from build123d import *

# Parameters (mm, degrees)
F1_DEPTH = 7.62
F2_R     = 2.54
F3_DEPTH = 25.4
F4_R     = 19.05
F4_R_2   = 8.89
F5_DEPTH = 25.4


with BuildPart() as f1:
    # F0 (on Top) → F1 (new body)
    with BuildSketch(Plane.XY):
        with BuildLine():
            ThreePointArc((-279.9174020173, 43.9496934414), (-263.0302165533, 39.4233371805), (-253.0018394569, 53.7445308008))
            ThreePointArc((-253.0018394569, 53.7445308008), (-262.5723411754, 67.8907101167), (-279.2635703278, 64.2696934414))
            Line((-279.2635703278, 64.2696934414), (-279.2635703278, 43.9496934414))
            Line((-279.2635703278, 43.9496934414), (-279.9174020173, 43.9496934414))
        make_face()
        with BuildLine():
            Line((-279.2635703278, 43.9496934414), (-279.2635703278, 64.2696934414))
            ThreePointArc((-279.2635703278, 64.2696934414), (-283.4739562591, 54.2346509123), (-279.9174020173, 43.9496934414))
            Line((-279.9174020173, 43.9496934414), (-279.2635703278, 43.9496934414))
        make_face()
        with BuildLine():
            ThreePointArc((-279.9174020173, 43.9496934414), (-283.4739562591, 54.2346509123), (-279.2635703278, 64.2696934414))
            Line((-279.2635703278, 64.2696934414), (-373.075891919, 64.2696934414))
            ThreePointArc((-373.075891919, 64.2696934414), (-370.1983304941, 59.5476620895), (-369.1951172447, 54.1096934414))
            ThreePointArc((-369.1951172447, 54.1096934414), (-370.1983304941, 48.6717247932), (-373.075891919, 43.9496934414))
            Line((-373.075891919, 43.9496934414), (-279.9174020173, 43.9496934414))
        make_face()
        with BuildLine():
            ThreePointArc((-369.1951172447, 54.1096934414), (-370.1983304941, 59.5476620895), (-373.075891919, 64.2696934414))
            Line((-373.075891919, 64.2696934414), (-373.2435703278, 64.2696934414))
            Line((-373.2435703278, 64.2696934414), (-373.2435703278, 43.9496934414))
            Line((-373.2435703278, 43.9496934414), (-373.075891919, 43.9496934414))
            ThreePointArc((-373.075891919, 43.9496934414), (-370.1983304941, 48.6717247932), (-369.1951172447, 54.1096934414))
        make_face()
        with BuildLine():
            Line((-373.2435703278, 64.2696934414), (-373.075891919, 64.2696934414))
            ThreePointArc((-373.075891919, 64.2696934414), (-399.6751172447, 54.1096934414), (-373.075891919, 43.9496934414))
            Line((-373.075891919, 43.9496934414), (-373.2435703278, 43.9496934414))
            Line((-373.2435703278, 43.9496934414), (-373.2435703278, 64.2696934414))
        make_face()
    extrude(amount=F1_DEPTH)

    # F2 (on face) → F3 (cut)
    with BuildSketch(Plane.XY.offset(7.62)):
        with Locations((-384.4351172447, 54.1096934414)):
            Circle(F2_R)
        with Locations((-268.2418394569, 53.7445308008)):
            Circle(F2_R)
    extrude(amount=-F3_DEPTH, mode=Mode.SUBTRACT)

    # F4 (on Top) → F5 (join)
    with BuildSketch(Plane.XY):
        with Locations((-404.0130972862, 38.6605933309)):
            Circle(F4_R)
        with Locations((-404.0130972862, 38.6605933309)):
            Circle(F4_R_2, mode=Mode.SUBTRACT)
    extrude(amount=F5_DEPTH)


solid = f1.part
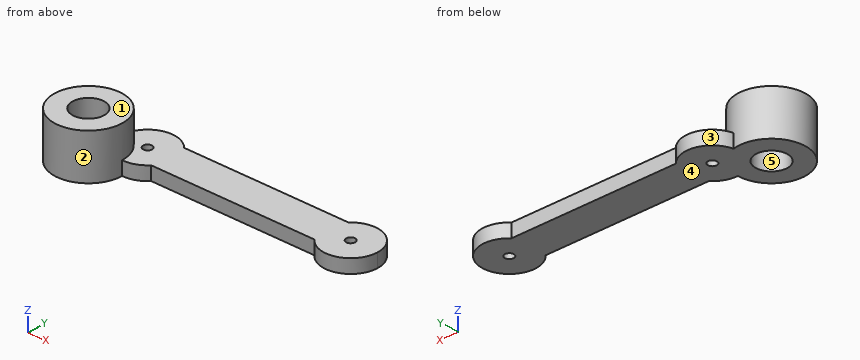
Input: part model. Units: mm. Frame: model coordinates. Face numbers are marked on the shaded views. A direction names the side the tool comes from. Round coordinates to 2 decimals unless told otherwise and drop trailing zeros. Write each loop counter-clockwise with the first axis right and the second up, starting at its lowest first coordinate (ties: lowest second). Pieces come first, ordered by that corner, then holes.
1) Ray query, L1, parallel to Y at x = -403.5, z = 5.5; L2, parallel to X at y = 40.5, z = 5.75; L3, parallel to Y at x = -365, z = 6. Return the intervals inside material, ascending.
2) Contact query for flat-ended pins moving along their axis: P1, Ø15.5, axis at x = -292.5, y = 50.5, coming from the +Z side; P2, Ø4, axis at y = 32.5, z = 14.5, coming from the -X side; P3, Ø4, axis at x = -324.5, z = 5.5, coming from the +Y side. Output: stop coordinate, or through.
3) Cut plane D-D (y = 23.5). Return the cut outline in (x, z).
4) Cut plane C-C (x = -336). Return the cut outline in (y, z), then the cut area to 3 significant figures.
5) Reachability of the marked faces 1 and 2 from +Z, -Z, +X, -X, +Y, -Y: full face, straight path, thin tool, end or side. Return the list, or none.
6) Draft query along X for the marked faces 3, 4 and 5. Return one class per face: pulls with the +X half, pulls with the -X half, needs draft (parallel to the pull), parting line crosses it, or undercut.
7) Cut plane A-A (y = 42.5). Return the cut outline in (x, z), then the cut area to 3 significant figures.
8) Cut plane B-B (z = 6). Return the cut outline in (x, y), then the cut area to 3 significant figures.
Geometry says:
1. L1: y = 19.62 to 29.79, 47.54 to 57.7
1. L2: x = -422.97 to -412.71, -395.32 to -377.58, -275.78 to -260.7
1. L3: y = 43.95 to 64.27
2. P1: stops at z = 7.62
2. P2: stops at x = -422.6
2. P3: stops at y = 64.27
3. outline: (-415.55, 0) - (-392.48, 0) - (-392.48, 25.4) - (-415.55, 25.4) - close
4. outline: (43.95, 0) - (64.27, 0) - (64.27, 7.62) - (43.95, 7.62) - close
4. area: 155 mm2
5. face 1: +Z, +X, -X, +Y, -Y
5. face 2: +Z
6. face 3: undercut
6. face 4: needs draft
6. face 5: undercut
7. outline: (-422.67, 0) - (-412.03, 0) - (-412.03, 25.4) - (-422.67, 25.4) - close; (-395.99, 0) - (-374.56, 0) - (-374.56, 7.62) - (-385.35, 7.62) - (-385.35, 25.4) - (-395.99, 25.4) - close; (-278.53, 0) - (-257.96, 0) - (-257.96, 7.62) - (-278.53, 7.62) - close
7. area: 780 mm2
8. outline: (-399.37, 57.14) arc R19.05 ccw (long way) to (-384.96, 38.88) arc R15.24 ccw to (-373.08, 43.95) - (-279.92, 43.95) arc R15.24 ccw (long way) to (-279.26, 64.27) - (-373.08, 64.27) arc R15.24 ccw to start; hole circle Ø17.78 at (-404.01, 38.66); hole circle Ø5.08 at (-384.44, 54.11); hole circle Ø5.08 at (-268.24, 53.74)
8. area: 3,950 mm2
